Geometry: final body of the model. Coordinates: model frame, mm. A direction names the side the tool comes from. Coordinates: 2 decimals unless noted, no trailing zeros. Write each loop counter-clockwise with the first axis right and the second up, starting at its lowest first coordinate (ties: lowest second). Pieces come first, ordered by that corner, then holes.
from build123d import *

# Parameters (mm, degrees)
SKETCH1_W                  = 200
SKETCH1_H                  = 83.89
WHEEL_STEERING_DUMMY_DEPTH = 340.92
SKETCH4_W                  = 30
SKETCH4_H                  = 20
SKETCH5_W                  = 20
SKETCH5_H                  = 30
SKETCH5_W_2                = 14
SKETCH5_H_2                = 24
MOUNT_TONGUE_DEPTH         = 35
SKETCH6_R                  = 5
MOUNT_HOLES_DEPTH          = 359.639177203
FILLET1_R                  = 7.5


with BuildPart() as part:
    # Sketch1 → Wheel & Steering Dummy (new body)
    with BuildSketch(Plane(origin=(0, 0, 0), x_dir=(1, 0, 0), z_dir=(0, 1, 0))):
        Rectangle(SKETCH1_W, SKETCH1_H)
    extrude(amount=-WHEEL_STEERING_DUMMY_DEPTH)

    # Mount Body: sweep along a path in Sketch3
    with BuildLine(Plane.XY) as mount_body_path:
        Line((0, 0), (0, 30))
        Line((0, 30), (58.328201005, 35.698665242))
    # Sketch4 → Mount Body (sweep)
    with BuildSketch(Plane(origin=(0, 0, 0), x_dir=(1, 0, 0), z_dir=(0, 1, 0))):
        Rectangle(SKETCH4_W, SKETCH4_H)
    sweep(path=mount_body_path.line, transition=Transition.RIGHT)

    # Sketch5 → Mount Tongue (cut)
    with BuildSketch(Plane(origin=(61.231488288, 5.982316409, 0), x_dir=(0, 0, -1), z_dir=(0.9952612526754551, 0.09723702444482771, 0))):
        with Locations((0, 29.85783758)):
            Rectangle(SKETCH5_W, SKETCH5_H)
        with Locations((0, 29.85783758)):
            Rectangle(SKETCH5_W_2, SKETCH5_H_2, mode=Mode.SUBTRACT)
    extrude(amount=-MOUNT_TONGUE_DEPTH, mode=Mode.SUBTRACT)

    # Sketch6 → Mount Holes (cut, through all)
    with BuildSketch(Plane.XY.offset(7)):
        with Locations((33.446669688, 33.26773963)):
            Circle(SKETCH6_R)
        with Locations((48.375588478, 34.726294997)):
            Circle(SKETCH6_R)
    extrude(amount=-MOUNT_HOLES_DEPTH, mode=Mode.SUBTRACT)

    # Fillet1
    fillet1_edges = [part.edges().sort_by_distance(p)[0] for p in [
        (-15, 43.605919649, 0),
        (15, 16.394080351, 0),
    ]]
    fillet(fillet1_edges, radius=FILLET1_R)


solid = part.part
Item 1: Set-up query: faces 1 (the flat face through (42.322, 22.078, 0.098)), 2 (the flat face through (23.474, 32.504, 9.029)), 3 (the flat face through (-15, 19, 0)), 4 (the flat face through (41, 34, 7)), 5 (the flat face through (5, 24, -10)). Return all of +Z, -Z, +X, -X, +Y, -Y with unobstructed straight access to the full face (end or side cutting, diameter ignored); none if empty.
Derived:
face 1: +Z, -Z, +X
face 2: none
face 3: +Z, -Z, -X, +Y
face 4: +Z, +X, +Y
face 5: -Z, +X, -X, +Y
Item 2: Material intervals for probe 1 along Y at (x, z) = (44, 0); probe 2 along Y at (x, z) = (-19.5, 33); probe 3 along X at (y, z) = (19.5, 4), sorted ascending.
Derived:
probe 1: y = -340.92 to 0, 22.24 to 32.31, 37.15 to 46.36
probe 2: y = -340.92 to 0
probe 3: x = -15 to 24.74
Item 3: Section A-A, the plane z = -16. Output: boundary loops of the cut face in (x, y), plus the area to 3 significant figures.
Derived:
outline: (-100, -340.92) - (100, -340.92) - (100, 0) - (-100, 0) - close
area: 68,200 mm2
Item 4: Pin query (flat end, axial travel): pin 1 (22 mm diameter, centred on x = 45, y = 34, fed in from -Z); pin 2 (5 mm diameter, centred on y = 3, z = 4, fed in from +X); pin 3 (22 mm diameter, centred on y = 18, z = -3, fed in from -X). Return the tip coordinate at first contact, or that it passes through.
Derived:
pin 1: stops at z = -7
pin 2: stops at x = 15
pin 3: stops at x = -15
Item 5: Section B-B, the plane x = -44.5. Output: boundary loops of the cut face in (y, z) (3 decimals).
Derived:
outline: (-340.92, -41.945) - (0, -41.945) - (0, 41.945) - (-340.92, 41.945) - close
